Input: part model. Units: mm. Frame: model coordinates. Coordinates: 2 decimals unless noted, no trailing zeros. Order: outer loops, then holes, each group sorted by start corner. A loop starts at its lowest first (then second) coordinate and runs counter-clockwise, first axis right, second up. Notation, with made-up numbers: (-19, 56) -> (36, 56) arc R16 cw to (36, 87) -> close; hole circle Ø10 at (10.25, 22). An arc over 180 degrees is marked (long way). Write each question's results on one line, items separated by ' | '.
```python
from build123d import *

# Parameters (mm, degrees)
BOSS_EXTRUDE1_DEPTH            = 6.35
F_1_1_DIAMETER_HOLE1_D         = 28.575
F_1_1_DIAMETER_HOLE1_DEPTH     = 25.4
F_1_1_DIAMETER_HOLE1_TIP       = 8.584796094
F_1_2_0_5_DIAMETER_HOLE1_D     = 12.7
F_1_2_0_5_DIAMETER_HOLE1_DEPTH = 25.4
F_1_2_0_5_DIAMETER_HOLE1_TIP   = 3.815464931


with BuildPart() as part:
    # Sketch1 → Boss-Extrude1 (new body)
    with BuildSketch(Plane.XY):
        with BuildLine():
            Line((-54.802639065, 48.60615919), (-11.597239065, 48.60615919))
            ThreePointArc((-11.597239065, 48.60615919), (-0.865369296, 45.295583298), (6.136456449, 36.514502629))
            Line((6.136456449, 36.514502629), (17.733695514, 6.958343439))
            ThreePointArc((17.733695514, 6.958343439), (12.633512254, -14.258221072), (-9.042758094, -16.766962338))
            Line((-9.042758094, -16.766962338), (-63.84539716, 12.789196852))
            ThreePointArc((-63.84539716, 12.789196852), (-73.273063161, 34.219412746), (-54.802639065, 48.60615919))
        make_face()
    extrude(amount=BOSS_EXTRUDE1_DEPTH)

    # 1 (1) Diameter Hole1
    with Locations(Plane.XY.offset(6.35)):
        with Locations((-54.802639065, 29.55615919), (-11.597239065, 29.55615919)):
            Hole(F_1_1_DIAMETER_HOLE1_D / 2, depth=F_1_1_DIAMETER_HOLE1_DEPTH)
            with Locations((0, 0, -(F_1_1_DIAMETER_HOLE1_DEPTH + F_1_1_DIAMETER_HOLE1_TIP / 2))):  # 118° drill point
                Cone(0, F_1_1_DIAMETER_HOLE1_D / 2, F_1_1_DIAMETER_HOLE1_TIP, mode=Mode.SUBTRACT)

    # 1/2 (0.5) Diameter Hole1
    with Locations(Plane.XY.offset(6.35)):
        with Locations((0, 0)):
            Hole(F_1_2_0_5_DIAMETER_HOLE1_D / 2, depth=F_1_2_0_5_DIAMETER_HOLE1_DEPTH)
            with Locations((0, 0, -(F_1_2_0_5_DIAMETER_HOLE1_DEPTH + F_1_2_0_5_DIAMETER_HOLE1_TIP / 2))):  # 118° drill point
                Cone(0, F_1_2_0_5_DIAMETER_HOLE1_D / 2, F_1_2_0_5_DIAMETER_HOLE1_TIP, mode=Mode.SUBTRACT)


solid = part.part
```
(1) Cut plane D-D, the plane x = -21.5. Return loops of the section in (y, z), plus the area to 3 significant figures.
Return value:
outline: (-10.05, 0) -> (19.26, 0) -> (19.26, 6.35) -> (-10.05, 6.35) -> close; (39.86, 0) -> (48.61, 0) -> (48.61, 6.35) -> (39.86, 6.35) -> close | area: 242 mm2
(2) Pin query (flat end, axial travel): P1, Ø17, axis at x = -11.6, y = 29.56, coming from the +Z side. Return the tip coordinate at first contact, or that it passes through.
Return value:
P1: through
(3) Mould query, pull axis Y, two halves, no side actions, for faces 1 (the face through (12.875, -14.04, 3.131)), 2 (the face through (-40.53, 30.18, 3.13)), 3 (the face through (-16, 15, 6.35)), 4 (the face through (1.38, -6.2, 3.13)). Classes: +Y half, -Y half, draft (parallel to the pull), parting line (faces both ways), or undercut.
Return value:
face 1: parting line | face 2: undercut | face 3: draft | face 4: undercut
(4) Cut plane B-B, the plane x = 0. Return loops of the section in (y, z), plus the area to 3 significant figures.
Return value:
outline: (-19.05, 0) -> (-6.35, 0) -> (-6.35, 6.35) -> (-19.05, 6.35) -> close; (6.35, 0) -> (21.21, 0) -> (21.21, 6.35) -> (6.35, 6.35) -> close; (37.9, 0) -> (44.67, 0) -> (44.67, 6.35) -> (37.9, 6.35) -> close | area: 218 mm2
(5) Cut plane C-C, the plane z = 4.25. Count the separate pieces of the cut face and the enclosed holes in it, plus the area to 3 significant figures.
Return value:
separate pieces: 1 | enclosed holes: 3 | area: 2,980 mm2
(6) Line query: line 1 along X through (y, z) = (24, 4.75); line 2 along Y through (x, z) = (0, 1.5); line 3 along X through (y, z) = (42.5, 5.75). Output: solid intervals per line, ascending. Write a range as from..to.
Return value:
line 1: -73.02..-67.97, -41.64..-24.76, 1.57..11.05 | line 2: -19.05..-6.35, 6.35..21.21, 37.9..44.67 | line 3: -68.78..-60.85, -48.75..-17.65, -5.55..2.38
(7) Cut plane A-A, the plane y = 34.5. Return loops of the section in (x, z), plus the area to 3 significant figures.
Return value:
outline: (-73.2, 0) -> (-68.21, 0) -> (-68.21, 6.35) -> (-73.2, 6.35) -> close; (-41.4, 0) -> (-25, 0) -> (-25, 6.35) -> (-41.4, 6.35) -> close; (1.81, 0) -> (6.93, 0) -> (6.93, 6.35) -> (1.81, 6.35) -> close | area: 168 mm2
